Here's how the part is built. I have some questions about the finished solid (model axes, mm). Face numbers are marked on the shaded views. A direction names the side the tool comes from. Round coordinates to 2 decimals unless told otherwise and drop trailing zeros. Order: outer loops, then holes, each group sorted by start corner. A loop starts at its lowest first (then second) coordinate and runs counter-clockwise, first axis right, second up. Notation, with made-up numbers: (1.5, 32.25) -> (10.5, 32.25) arc R27 ccw to (10.5, 67.25) -> close; hole circle Ø3 at (15, -26). An arc over 180 degrees is marked (long way). Use a Markdown table: item, result. Add a question column.
(1) I want a section at C-C, the plane x = 5.5. Please give me the cut outline in (y, z).
(2) Thinking about a two-plate mould opening in Y: for the marked faces 1, 2 and 3, which applies, pulls with the +Y half, pulls with the -Y half, needs draft (parallel to the pull), parting line crosses it, or undercut?
(3) I'm going to push flat-ended pins straight in: P1, Ø2, axis at y = 5, z = 9, coming from the -X side; P2, Ø8, axis at y = -3.5, z = 8, coming from the -X side; P3, Ø1.6, axis at x = 9, y = -11, coming from the +Z side. Where does each tip first touch, or does it pass through?
(4) I want a section at A-A, the plane y = 0. Please give me the cut outline in (x, z).
(5) If I drill on probe 1 along Y at (x, z) = (10.95, 12.5); probe 2 along Z at (x, y) = (11.15, 0); probe 3 along X at (y, z) = (3, 6.25), over which ranges is the centre line in solid material (lowest first)?
(6) I want a section at B-B, the plane z = 7.5. Please give me the cut outline in (x, y) (3 decimals).
(7) On a 3-axis mill with a long thin cutter (end or side, diameter ignored), from which of +Z, -Z, +X, -X, +Y, -Y can I reach the whole of each face in a straight line? I mean the marked faces 4, 5 and 6. Say none if no direction works.
(8) I want a section at D-D, the plane y = -7.5. Please give me the cut outline in (x, z).
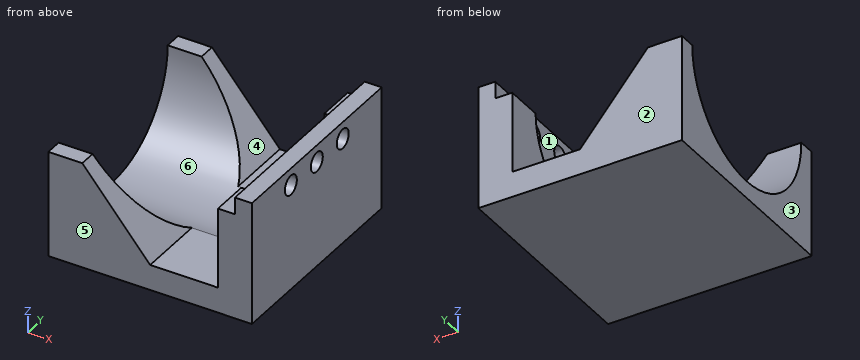
Solid Edge part; units mm, degrees
sketch "Sketch1" plane through (0, -12.5, 0) normal (0, -1, 0) x (1, 0, 0)
  line L0 (-12, 0) -> (-12, 12.5)
  line L1 (-12, 12.5) -> (-8, 12.5)
  line L2 (-8, 12.5) -> (0, 3)
  line L3 (0, 3) -> (8, 3)
  line L4 (8, 3) -> (8, 12.5)
  line L5 (8, 12.5) -> (10, 12.5)
  line L6 (10, 12.5) -> (10, 14.5)
  line L7 (10, 14.5) -> (12, 14.5)
  line L8 (12, 14.5) -> (12, 0)
  line L9 (-12, 0) -> (12, 0)
extrude "Protrusion1" add sketch "Sketch1" against normal up to vertex (25 mm away)
sketch "Sketch2" plane through (-12, 0, 6.25) normal (-1, 0, 0) x (0, -1, 0)
  circle A0 centre (0, 6.25) radius 10.5
extrude "Cutout1" cut sketch "Sketch2" against normal up to vertex (20 mm away)
sketch "Sketch3" plane through (8, 0, 7.75) normal (-1, 0, 0) x (0, -1, 0)
  circle A0 centre (0, 4.75) radius 8
extrude "Cutout2" cut sketch "Sketch3" against normal blind 2
hole "Hole_4" at (12, 5, 12.5) direction (-1, 0, 0) diameter 2.3 end up to next
hole "Hole1" at (12, 0, 12.5) direction (-1, 0, 0) diameter 2.3 end up to next
hole "Hole2" at (12, -5, 12.5) direction (-1, 0, 0) diameter 2.3 end up to next
Taken from the geometry:
| question | item | result |
|---|---|---|
| 1 | outline | (-12.5, 0) -> (12.5, 0) -> (12.5, 3) -> (4.47, 3) arc R10.5 cw to (-4.47, 3) -> (-12.5, 3) -> close |
| 2 | face 1 | undercut |
| 2 | face 2 | pulls with the +Y half |
| 2 | face 3 | needs draft |
| 3 | P1 | stops at x = 10 |
| 3 | P2 | stops at x = 8 |
| 3 | P3 | stops at z = 12.5 |
| 4 | outline | (-12, 0) -> (12, 0) -> (12, 11.35) -> (10, 11.35) -> (10, 4.5) -> (8, 4.5) -> (8, 2) -> (-12, 2) -> close; (10, 13.65) -> (12, 13.65) -> (12, 14.5) -> (10, 14.5) -> close |
| 5 | probe 1 | y = -12.5 to -6.15, -3.85 to -1.15, 1.15 to 3.85, 6.15 to 12.5 |
| 5 | probe 2 | z = 0 to 11.35, 13.65 to 14.5 |
| 5 | probe 3 | x = 10 to 12 |
| 6 | outline | (-12, -12.5) -> (-3.789, -12.5) -> (-3.789, -9.233) -> (-12, -9.233) -> close; (-12, 9.233) -> (-3.789, 9.233) -> (-3.789, 12.5) -> (-12, 12.5) -> close; (8, -12.5) -> (12, -12.5) -> (12, 12.5) -> (8, 12.5) -> (8, 6.245) -> (10, 6.245) -> (10, -6.245) -> (8, -6.245) -> close |
| 7 | face 4 | +Z, +Y, -Y |
| 7 | face 5 | +Z, -Z, +X, -X, -Y |
| 7 | face 6 | +Z, -X |
| 8 | outline | (-12, 0) -> (12, 0) -> (12, 14.5) -> (10, 14.5) -> (10, 9.72) -> (8, 9.72) -> (8, 3) -> (0, 3) -> (-1.81, 5.15) -> (-12, 5.15) -> close |
